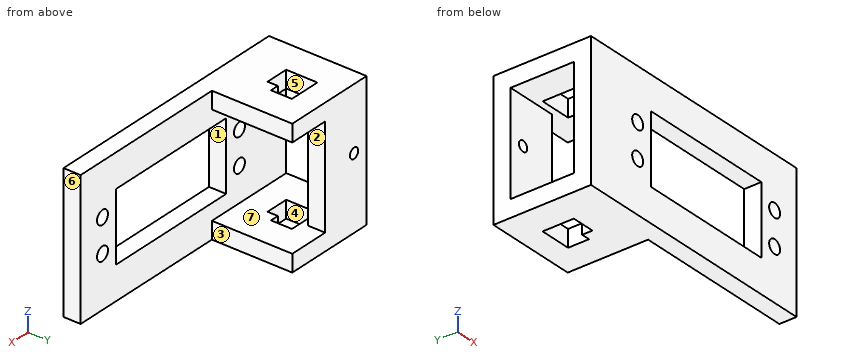
from build123d import *

# Parameters (mm, degrees)
SKETCH1_R           = 2
SKETCH1_W           = 40
SKETCH1_H           = 19.81
BOSS_EXTRUDE1_DEPTH = 5
SKETCH2_W           = 23.106523906
SKETCH2_H           = 5
BOSS_EXTRUDE2_DEPTH = 18.45
SKETCH3_W           = 23.106523906
SKETCH3_H           = 5
BOSS_EXTRUDE3_DEPTH = 39.55
CUT_EXTRUDE1_START  = -39.55
CUT_EXTRUDE1_DEPTH  = 39.55
SKETCH6_W           = 12
SKETCH6_H           = 29.55
CUT_EXTRUDE2_DEPTH  = 23.45
CUT_EXTRUDE3_START  = -39.55
CUT_EXTRUDE3_DEPTH  = 39.55
SKETCH9_W           = 39.55
SKETCH9_H           = 28.45
SKETCH9_W_2         = 29.55
SKETCH9_H_2         = 18.45
BOSS_EXTRUDE4_DEPTH = 4
SKETCH11_W          = 39.55
SKETCH11_H          = 5
BOSS_EXTRUDE5_DEPTH = 3
SKETCH12_W          = 40.3
SKETCH12_H          = 20.11
SKETCH12_W_2        = 40
SKETCH12_H_2        = 19.81
CUT_EXTRUDE4_DEPTH  = 5
SKETCH13_R          = 1.5
CUT_EXTRUDE5_DEPTH  = 5


with BuildPart() as part:
    # Sketch1 → Boss-Extrude1 (new body)
    with BuildSketch(Plane(origin=(0, 0, 0), x_dir=(1, 0, 0), z_dir=(0, 1, 0))):
        Polygon((32, -9.9), (32, 10.1), (32, 18.775), (32, 19.775), (31, 19.775), (-13.05, 19.775), (-27, 19.775), (-36.05, 19.775), (-36.05, -19.775), (-27, -19.775), (-13.05, -19.775), (31, -19.775), (32, -19.775), (32, -18.775), align=None)
        with Locations(Location((-23, -4.82, 0), (0, 0, 270))):
            Circle(SKETCH1_R, mode=Mode.SUBTRACT)
        with Locations(Location((-23, 4.83, 0), (0, 0, 270))):
            Circle(SKETCH1_R, mode=Mode.SUBTRACT)
        with Locations(Location((27, -4.82, 0), (0, 0, 90))):
            Circle(SKETCH1_R, mode=Mode.SUBTRACT)
        with Locations(Location((27, 4.83, 0), (0, 0, 90))):
            Circle(SKETCH1_R, mode=Mode.SUBTRACT)
        with Locations((2, 0.005)):
            Rectangle(SKETCH1_W, SKETCH1_H, mode=Mode.SUBTRACT)
    extrude(amount=BOSS_EXTRUDE1_DEPTH)

    # Sketch2 → Boss-Extrude2 (add)
    with BuildSketch(Plane(origin=(0, 5, 0), x_dir=(1, 0, 0), z_dir=(0, 1, 0))):
        with Locations((-24.496738047, -17.275)):
            Rectangle(SKETCH2_W, SKETCH2_H)
        with Locations((-24.496738047, 17.275)):
            Rectangle(SKETCH2_W, SKETCH2_H)
    extrude(amount=BOSS_EXTRUDE2_DEPTH)

    # Sketch3 → Boss-Extrude3 (add)
    with BuildSketch(Plane.XY.offset(19.775)):
        with Locations((-24.496738047, 25.95)):
            Rectangle(SKETCH3_W, SKETCH3_H)
    extrude(amount=-BOSS_EXTRUDE3_DEPTH)

    # Sketch4 → Cut-Extrude1 (cut)
    with BuildSketch(Plane.XY.offset(19.775).offset(CUT_EXTRUDE1_START)):
        Polygon((-24.05, 21.45), (-30.75, 21.45), (-30.75, 15.45), (-30.75, 12.45), (-24.05, 12.45), (-24.05, 15.45), (-21.55, 15.45), (-21.55, 21.45), align=None)
    extrude(amount=CUT_EXTRUDE1_DEPTH, mode=Mode.SUBTRACT)

    # Sketch6 → Cut-Extrude2 (cut)
    with BuildSketch(Plane(origin=(0, 5, 0), x_dir=(1, 0, 0), z_dir=(0, 1, 0))):
        with Locations((-18.943476094, 0)):
            Rectangle(SKETCH6_W, SKETCH6_H)
    extrude(amount=CUT_EXTRUDE2_DEPTH, mode=Mode.SUBTRACT)

    # Sketch7 → Cut-Extrude3 (cut)
    with BuildSketch(Plane.XY.offset(19.775).offset(CUT_EXTRUDE3_START)):
        Polygon((-24.05, 21.5), (-30.8, 21.5), (-30.8, 15.45), (-30.8, 12.4), (-24, 12.4), (-24, 15.4), (-21.5, 15.4), (-21.5, 21.5), align=None)
        Polygon((-24.05, 21.45), (-30.75, 21.45), (-30.75, 15.45), (-30.75, 12.45), (-24.05, 12.45), (-24.05, 15.45), (-21.55, 15.45), (-21.55, 21.45), align=None, mode=Mode.SUBTRACT)
    extrude(amount=CUT_EXTRUDE3_DEPTH, mode=Mode.SUBTRACT)

    # Sketch9 → Boss-Extrude4 (add)
    with BuildSketch(Plane.ZY.offset(36.05)):
        with Locations((0, 14.225)):
            Rectangle(SKETCH9_W, SKETCH9_H)
        with Locations((0, 14.225)):
            Rectangle(SKETCH9_W_2, SKETCH9_H_2, mode=Mode.SUBTRACT)
    extrude(amount=BOSS_EXTRUDE4_DEPTH)

    # Sketch11 → Boss-Extrude5 (add)
    with BuildSketch(Plane(origin=(32, 0, 0), x_dir=(0, 0, -1), z_dir=(1, 0, 0))):
        with Locations((0, 2.5)):
            Rectangle(SKETCH11_W, SKETCH11_H)
    extrude(amount=BOSS_EXTRUDE5_DEPTH)

    # Sketch12 → Cut-Extrude4 (cut)
    with BuildSketch(Plane(origin=(0, 5, 0), x_dir=(1, 0, 0), z_dir=(0, 1, 0))):
        with Locations((2, 0.005)):
            Rectangle(SKETCH12_W, SKETCH12_H)
        with Locations((2, 0.005)):
            Rectangle(SKETCH12_W_2, SKETCH12_H_2, mode=Mode.SUBTRACT)
    extrude(amount=-CUT_EXTRUDE4_DEPTH, mode=Mode.SUBTRACT)

    # Sketch13 → Cut-Extrude5 (cut)
    with BuildSketch(Plane(origin=(0, 28.45, 0), x_dir=(1, 0, 0), z_dir=(0, 1, 0))):
        with Locations(Location((-35.49673805, -1.395, 0), (0, 0, 270))):
            Circle(SKETCH13_R)
    extrude(amount=-CUT_EXTRUDE5_DEPTH, mode=Mode.SUBTRACT)


solid = part.part
Geometry check sheet. Reference: the model listing, model coordinates, mm. Face numbers are marked on the shaded views. A direction names the side the tool comes from. Round coordinates to 2 decimals unless told otherwise and drop trailing zeros. Order: outer loops, then holes, each group sorted by start corner. A loop starts at its lowest first (then second) coordinate and runs counter-clockwise, first axis right, second up. Notation, with made-up numbers: M -26,-32 L 24,-32 A19 cw 24,0 Z; hole C 37.5,1 d8. An arc over 180 degrees is marked long. Answer in a Markdown table with one row per item. Add a question column.
Item 1: Material ranges on L1, parallel to X at y = 1.2, z = 4.82; L2, parallel to Z at x = -23, y = 1.8 (3 decimals); L3, parallel to Z at x = -21, y = 10.75 (3 decimals), recorded low to high. Write a range as [from, to].
Item 2: Sectioned sample at C-C, the plane x = 27. Enter the section's corners in (y, z) (3 decimals).
Item 3: Sectioned sample at B-B, the plane z = 13. Enter the section's corners in (x, y).
Item 4: Sectioned sample at D-D, the plane y = 17.25. Enter the section's corners in (x, z) (3 decimals).
Item 5: Draft check along X on the marked faces 4, 5, 6 and 7. Enter one of: released by +X, released by -X, zero draft, split by the parting line, or undercut.
Item 6: Depth check by flat-ended pin: pin 1 Ø4 at (y, z) = (16, -16.5) entering from +X; pin 2 Ø1 at (x, z) = (-18, 11.5) entering from +Y; pin 3 Ø2.5 at (y, z) = (27, 2) entering from +X. Enter the tip coordinate at first touch or a pass-through.
Item 7: Sectioned sample at A-A, the plane x = -26. Enter the section's corners in (y, z) (3 decimals).
Item 8: Set-up check for the marked faces 1, 2 and 3: record each of +Z, -Z, +X, -X, +Y, -Y from which the full face is reachable in a straight line by a thin tool's end or side.
Filled in:
| question | item | result |
|---|---|---|
| 1 | L1 | x = [-40.05, -25], [-21, -18.15], [22.15, 25], [29, 35] |
| 1 | L2 | z = [-19.775, -6.83], [-2.83, 2.82], [6.82, 19.775] |
| 1 | L3 | z = [-19.775, -14.775], [14.775, 19.775] |
| 2 | outline | M 0,-19.775 L 5,-19.775 L 5,-6.83 L 0,-6.83 Z; M 0,-2.83 L 5,-2.83 L 5,2.82 L 0,2.82 Z; M 0,6.82 L 5,6.82 L 5,19.775 L 0,19.775 Z |
| 3 | outline | M -40.05,0 L 35,0 L 35,5 L -40.05,5 Z; M -40.05,23.45 L -24.94,23.45 L -24.94,28.45 L -40.05,28.45 Z |
| 4 | outline | M -40.05,-19.775 L -30.8,-19.775 L -30.8,-14.775 L -40.05,-14.775 Z; M -40.05,14.775 L -30.8,14.775 L -30.8,19.775 L -40.05,19.775 Z; M -21.5,-19.775 L -12.943,-19.775 L -12.943,-14.775 L -21.5,-14.775 Z; M -21.5,14.775 L -12.943,14.775 L -12.943,19.775 L -21.5,19.775 Z |
| 5 | face 4 | undercut |
| 5 | face 5 | undercut |
| 5 | face 6 | released by +X |
| 5 | face 7 | zero draft |
| 6 | pin 1 | stops at x = -12.94 |
| 6 | pin 2 | stops at y = 5 |
| 6 | pin 3 | stops at x = -24.94 |
| 7 | outline | M 0,-19.775 L 12.4,-19.775 L 12.4,-14.775 L 5,-14.775 L 5,14.775 L 12.4,14.775 L 12.4,19.775 L 0,19.775 Z; M 21.5,-19.775 L 28.45,-19.775 L 28.45,19.775 L 21.5,19.775 L 21.5,14.775 L 23.45,14.775 L 23.45,-14.775 L 21.5,-14.775 Z |
| 8 | face 1 | +Y, -Y |
| 8 | face 2 | +X, +Y |
| 8 | face 3 | +Z, -Z, +X, +Y |
